The listing builds one solid part. Answer for the finished solid, in the listing's coordinates (mm). A direction names the side the tool comes from. Coordinates: 2 decimals unless noted, no trailing zeros. Order: outer loops, then holes, each group sorted by start corner. A loop starts at its lowest first (then second) coordinate and runs counter-clockwise, first axis right, second up. Notation, with made-up numbers: (-13, -1.5) -> (11, -1.5) arc R19 cw to (11, 5.5) -> close; hole circle Ø5 at (63, -2.75). An arc over 180 degrees is marked (long way). Answer in a Markdown table with one row per item. Add a question column.
```python
from build123d import *

# Parameters (mm, degrees)
F1_DEPTH  = 14
F2_W      = 102
F2_H      = 10
F3_DEPTH  = 65
F4_R      = 20
F6_DEPTH  = 10
F7_R      = 7
F8_DEPTH  = 14
F9_R      = 7
F10_DEPTH = 14
F12_DEPTH = 58


with BuildPart() as f1:
    # F0 (on Top) → F1 (new body)
    with BuildSketch(Plane.XY):
        with BuildLine():
            ThreePointArc((-78.572579, -32.704081), (-77.108113, -36.239615), (-73.572579, -37.704081))
            Line((-73.572579, -37.704081), (48.427421, -37.704081))
            ThreePointArc((48.427421, -37.704081), (51.962955, -36.239615), (53.427421, -32.704081))
            Line((53.427421, -32.704081), (53.427421, 15.295919))
            ThreePointArc((53.427421, 15.295919), (51.962955, 18.831453), (48.427421, 20.295919))
            Line((48.427421, 20.295919), (-73.572579, 20.295919))
            ThreePointArc((-73.572579, 20.295919), (-77.108113, 18.831453), (-78.572579, 15.295919))
            Line((-78.572579, 15.295919), (-78.572579, -32.704081))
        make_face()
    extrude(amount=F1_DEPTH)

    # F2 (on face) → F3 (join)
    with BuildSketch(Plane.XY.offset(14)):
        with Locations((-12.572579, 15.295919)):
            Rectangle(F2_W, F2_H)
    extrude(amount=F3_DEPTH)

    # F4
    f4_edges = [f1.edges().sort_by_distance(p)[0] for p in [
        (-63.572579, 15.295919, 79),
        (38.427421, 15.295919, 79),
    ]]
    fillet(f4_edges, radius=F4_R)

    # F5 (on face) → F6 (cut)
    with BuildSketch(Plane.XZ.offset(-10.295919)):
        with BuildLine():
            Line((18.427421, 69), (-43.572579, 69))
            ThreePointArc((-43.572579, 69), (-53.572579, 59), (-43.572579, 49))
            Line((-43.572579, 49), (18.427421, 49))
            ThreePointArc((18.427421, 49), (28.427421, 59), (18.427421, 69))
        make_face()
    extrude(amount=-F6_DEPTH, mode=Mode.SUBTRACT)

    # F7 (on face) → F8 (cut)
    with BuildSketch(Plane.XY.offset(14)):
        with Locations((-62.572579, -8.704081)):
            Circle(F7_R)
    extrude(amount=-F8_DEPTH, mode=Mode.SUBTRACT)

    # F9 (on face) → F10 (cut)
    with BuildSketch(Plane.XY.offset(14)):
        with Locations((37.427421, -8.704081)):
            Circle(F9_R)
    extrude(amount=-F10_DEPTH, mode=Mode.SUBTRACT)

    # F11 (on face) → F12 (join)
    with BuildSketch(Plane.XY.offset(14)):
        Polygon((-50.072579, -37.704081), (-12.572579, -37.704081), (24.927421, -37.704081), (24.927421, -27.704081), (-50.072579, -27.704081), align=None)
    extrude(amount=F12_DEPTH)


solid = f1.part
```
Q1. Given pin 1 (12.5 mm diameter, centred on x = -62.57, y = -8.7, fed in from -Z) (1 decimal); pin 2 (8 mm diameter, centred on y = 13, z = 39, fed in from +X); pin 3 (11 mm diameter, centred on y = -34, z = 48, fed in from +X); pin 4 (11 mm diameter, centred on y = -35, z = 50.5, fed in from -X), each flat-ended and moving along its own axis, determine where each tip first touches the part or whether it passes through.
Q2. A cutting plane is placed at C-C (z = 11.5). Determine the outline of the cut face in (x, y).
Q3. A cutting plane is placed at B-B (x = -16). Determine the outline of the cut face in (y, z).
Q4. Determine the mould class of faces 1 (the face through (28.425, 15.226, 58.78)), 2 (the face through (-13, -37.704, 27)), 3 (the face through (-13, 15, 79)) for opening direction Z: +Z half, -Z half, draft (parallel to the pull), parting line (faces both ways), or undercut.
Q5. For faces 4 (the face through (-12, -27.704, 43)), 5 (the face through (-13, 15, 49)), 6 (the face through (24.927, -33, 43)), determine the directions among +Z, -Z, +X, -X, +Y, -Y from which every point of the face is accessible in a straight line to the end or side of a thin tool.
Q6. Straight lines are drawn through the part: line 1 (Y direction, x = -12.5, z = 44); line 2 (X direction, y = -7.5, z = 13.5); line 3 (Z direction, x = -6, y = 13.5). For each, find the intervals that lie inside material, in ascending order.
Q7. A cutting plane is placed at A-A (z = 30.5). Determine the outline of the cut face in (x, y), then the cut area to 3 significant figures.
Returned:
| question | item | result |
|---|---|---|
| 1 | pin 1 | passes through |
| 1 | pin 2 | stops at x = 38.43 |
| 1 | pin 3 | stops at x = 24.93 |
| 1 | pin 4 | stops at x = -50.07 |
| 2 | outline | (-78.57, -32.7) arc R5 ccw to (-73.57, -37.7) -> (48.43, -37.7) arc R5 ccw to (53.43, -32.7) -> (53.43, 15.3) arc R5 ccw to (48.43, 20.3) -> (-73.57, 20.3) arc R5 ccw to (-78.57, 15.3) -> close; hole circle Ø14 at (-62.57, -8.7); hole circle Ø14 at (37.43, -8.7) |
| 3 | outline | (-37.7, 0) -> (20.3, 0) -> (20.3, 49) -> (10.3, 49) -> (10.3, 14) -> (-27.7, 14) -> (-27.7, 72) -> (-37.7, 72) -> close; (10.3, 69) -> (20.3, 69) -> (20.3, 79) -> (10.3, 79) -> close |
| 4 | face 1 | undercut |
| 4 | face 2 | draft |
| 4 | face 3 | +Z half |
| 5 | face 4 | +Z, +X, -X |
| 5 | face 5 | +Y |
| 5 | face 6 | +Z, +X, -Y |
| 6 | line 1 | y = -37.7 to -27.7, 10.3 to 20.3 |
| 6 | line 2 | x = -78.57 to -69.47, -55.68 to 30.53, 44.32 to 53.43 |
| 6 | line 3 | z = 0 to 49, 69 to 79 |
| 7 | outline | (-63.57, 10.3) -> (38.43, 10.3) -> (38.43, 20.3) -> (-63.57, 20.3) -> close; (-50.07, -37.7) -> (24.93, -37.7) -> (24.93, -27.7) -> (-50.07, -27.7) -> close |
| 7 | area | 1,770 mm² |
